```python
from build123d import *

# Parameters (mm, degrees)
ESQUISSE1_W              = 120
ESQUISSE1_H              = 160
BOSS_EXTRU_1_DEPTH       = 40
ESQUISSE2_W              = 110
ESQUISSE2_H              = 150
ENL_V_MAT_EXTRU_1_DEPTH  = 35
CONG_1_R                 = 10
CONG_2_R                 = 10
CONG_3_R                 = 10
ESQUISSE3_R              = 2.5
BOSS_EXTRU_2_DEPTH       = 2.5
CONG_4_R                 = 2.5
ESQUISSE4_R              = 3
ENL_V_MAT_EXTRU_2_DEPTH  = 35
ESQUISSE5_W              = 11
ESQUISSE5_H              = 52
ENL_V_MAT_EXTRU_3_DEPTH  = 2
ESQUISSE6_W              = 52
ESQUISSE6_H              = 11
ENL_V_MAT_EXTRU_4_DEPTH  = 2
ESQUISSE8_W              = 22
ESQUISSE8_H              = 27
ENL_V_MAT_EXTRU_6_DEPTH  = 5
ESQUISSE10_R             = 1
ENL_V_MAT_EXTRU_7_DEPTH  = 4
ESQUISSE11_W             = 10
ESQUISSE11_H             = 10
ENL_V_MAT_EXTRU_8_DEPTH  = 201.062490237
ESQUISSE12_W             = 10
ESQUISSE12_H             = 5.85
ENL_V_MAT_EXTRU_9_DEPTH  = 3
ESQUISSE13_W             = 22
ESQUISSE13_H             = 27
ENL_V_MAT_EXTRU_10_DEPTH = 1
ESQUISSE14_R             = 1
ENL_V_MAT_EXTRU_11_DEPTH = 6
ESQUISSE15_R             = 5
ENL_V_MAT_EXTRU_12_DEPTH = 197.979694385
ESQUISSE16_W             = 22
ESQUISSE16_H             = 17
ENL_V_MAT_EXTRU_13_DEPTH = 2
ESQUISSE17_W             = 26
ESQUISSE17_H             = 22
ENL_V_MAT_EXTRU_14_DEPTH = 2
ESQUISSE18_W             = 26
ESQUISSE18_H             = 22
ENL_V_MAT_EXTRU_15_DEPTH = 2


with BuildPart() as part:
    # Esquisse1 → Boss.-Extru.1 (new body)
    with BuildSketch(Plane(origin=(0, 0, 0), x_dir=(1, 0, 0), z_dir=(0, 1, 0))):
        with Locations((60, 80)):
            Rectangle(ESQUISSE1_W, ESQUISSE1_H)
    extrude(amount=BOSS_EXTRU_1_DEPTH)

    # Esquisse2 → Enlèv. mat.-Extru.1 (cut)
    with BuildSketch(Plane(origin=(0, 40, 0), x_dir=(1, 0, 0), z_dir=(0, 1, 0))):
        with Locations((65, 75)):
            Rectangle(ESQUISSE2_W, ESQUISSE2_H)
    extrude(amount=-ENL_V_MAT_EXTRU_1_DEPTH, mode=Mode.SUBTRACT)

    # Congé1
    cong_1_edges = [part.edges().sort_by_distance(p)[0] for p in [
        (60, 0, -160),
    ]]
    fillet(cong_1_edges, radius=CONG_1_R)

    # Congé2
    cong_2_edges = [part.edges().sort_by_distance(p)[0] for p in [
        (0, 0, -75),
        (0, 2.928932188, -157.071067812),
        (0, 25, -160),
    ]]
    fillet(cong_2_edges, radius=CONG_2_R)

    # Congé3
    cong_3_edges = [part.edges().sort_by_distance(p)[0] for p in [
        (10, 22.5, -150),
    ]]
    fillet(cong_3_edges, radius=CONG_3_R)

    # Esquisse3 → Boss.-Extru.2 (add)
    with BuildSketch(Plane.XZ):
        with Locations(Location((30, -130, 0), (0, 0, 270))):
            Circle(ESQUISSE3_R)
    extrude(amount=BOSS_EXTRU_2_DEPTH)

    # Congé4
    cong_4_edges = [part.edges().sort_by_distance(p)[0] for p in [
        (30, -2.5, -127.5),
    ]]
    fillet(cong_4_edges, radius=CONG_4_R - 0.0001)  # a hair under: the kernel refuses the full size

    # Esquisse4 → Enlèv. mat.-Extru.2 (cut)
    with BuildSketch(Plane(origin=(0, 40, 0), x_dir=(1, 0, 0), z_dir=(0, 1, 0))):
        with Locations(Location((8, 152, 0), (0, 0, 270))):
            Circle(ESQUISSE4_R)
    extrude(amount=-ENL_V_MAT_EXTRU_2_DEPTH, mode=Mode.SUBTRACT)

    # Esquisse5 → Enlèv. mat.-Extru.3 (cut)
    with BuildSketch(Plane(origin=(0, 5, 0), x_dir=(1, 0, 0), z_dir=(0, 1, 0))):
        with Locations((114.5, 75)):
            Rectangle(ESQUISSE5_W, ESQUISSE5_H)
    extrude(amount=-ENL_V_MAT_EXTRU_3_DEPTH, mode=Mode.SUBTRACT)

    # Esquisse6 → Enlèv. mat.-Extru.4 (cut)
    with BuildSketch(Plane(origin=(0, 5, 0), x_dir=(1, 0, 0), z_dir=(0, 1, 0))):
        with Locations((65, 5.5)):
            Rectangle(ESQUISSE6_W, ESQUISSE6_H)
    extrude(amount=-ENL_V_MAT_EXTRU_4_DEPTH, mode=Mode.SUBTRACT)

    # Esquisse8 → Enlèv. mat.-Extru.6 (cut)
    with BuildSketch(Plane.XY.offset(-150)):
        with Locations((41, 22.5)):
            Rectangle(ESQUISSE8_W, ESQUISSE8_H)
    extrude(amount=-ENL_V_MAT_EXTRU_6_DEPTH, mode=Mode.SUBTRACT)

    # Esquisse10 → Enlèv. mat.-Extru.7 (cut)
    with BuildSketch(Plane.XY.offset(-155)):
        with Locations((41, 32.75)):
            Circle(ESQUISSE10_R)
        with Locations((41, 12.25)):
            Circle(ESQUISSE10_R)
    extrude(amount=-ENL_V_MAT_EXTRU_7_DEPTH, mode=Mode.SUBTRACT)

    # Esquisse11 → Enlèv. mat.-Extru.8 (cut, through all)
    with BuildSketch(Plane.XY.offset(-155)):
        with Locations((41, 25.75)):
            Rectangle(ESQUISSE11_W, ESQUISSE11_H)
    extrude(amount=-ENL_V_MAT_EXTRU_8_DEPTH, mode=Mode.SUBTRACT)

    # Esquisse12 → Enlèv. mat.-Extru.9 (cut)
    with BuildSketch(Plane.XY.offset(-155)):
        with Locations((41, 17.825)):
            Rectangle(ESQUISSE12_W, ESQUISSE12_H)
    extrude(amount=-ENL_V_MAT_EXTRU_9_DEPTH, mode=Mode.SUBTRACT)

    # Esquisse13 → Enlèv. mat.-Extru.10 (cut)
    with BuildSketch(Plane.XY.offset(-150)):
        with Locations((78, 22.5)):
            Rectangle(ESQUISSE13_W, ESQUISSE13_H)
    extrude(amount=-ENL_V_MAT_EXTRU_10_DEPTH, mode=Mode.SUBTRACT)

    # Esquisse14 → Enlèv. mat.-Extru.11 (cut)
    with BuildSketch(Plane.XY.offset(-151)):
        with Locations((78, 32.5)):
            Circle(ESQUISSE14_R)
        with Locations((78, 12.5)):
            Circle(ESQUISSE14_R)
    extrude(amount=-ENL_V_MAT_EXTRU_11_DEPTH, mode=Mode.SUBTRACT)

    # Esquisse15 → Enlèv. mat.-Extru.12 (cut, through all)
    with BuildSketch(Plane.XY.offset(-151)):
        with Locations((78, 22.5)):
            Circle(ESQUISSE15_R)
    extrude(amount=-ENL_V_MAT_EXTRU_12_DEPTH, mode=Mode.SUBTRACT)

    # Esquisse16 → Enlèv. mat.-Extru.13 (cut)
    with BuildSketch(Plane.XY.offset(-151)):
        with Locations((78, 22.5)):
            Rectangle(ESQUISSE16_W, ESQUISSE16_H)
    extrude(amount=-ENL_V_MAT_EXTRU_13_DEPTH, mode=Mode.SUBTRACT)

    # Esquisse17 → Enlèv. mat.-Extru.14 (cut)
    with BuildSketch(Plane.XY.offset(-150)):
        with Locations((107, 22.5)):
            Rectangle(ESQUISSE17_W, ESQUISSE17_H)
    extrude(amount=-ENL_V_MAT_EXTRU_14_DEPTH, mode=Mode.SUBTRACT)

    # Esquisse18 → Enlèv. mat.-Extru.15 (cut)
    with BuildSketch(Plane(origin=(10, 0, 0), x_dir=(0, 0, -1), z_dir=(1, 0, 0))):
        with Locations((13, 22.5)):
            Rectangle(ESQUISSE18_W, ESQUISSE18_H)
    extrude(amount=-ENL_V_MAT_EXTRU_15_DEPTH, mode=Mode.SUBTRACT)


solid = part.part
```
Can you work these out from the model? Positions are in its coordinate system, mm. A direction names the side the tool comes from. Round coordinates to 2 decimals unless told otherwise and drop trailing zeros. Order: outer loops, then holes, each group sorted by start corner. A loop starts at its lowest first (then second) coordinate and runs counter-clockwise, first axis right, second up. Notation, with made-up numbers: (-39, 77) -> (-5, 77) arc R28 cw to (-5, 95) -> close; hole circle Ø3 at (23, -1). An arc over 180 degrees is marked (long way). Return JSON: item names as keys, results as strings. Group by question number.
1. If we section it at A-A, the plane y = 22.5: Count the separate pieces of the cut face and the enclosed holes in it, then the cut area to 3 significant figures.
2. We'd pull the mould along Z, two halves only. Please class faces 5 (the face through (82.619, 20.585, -156.451)), 6 (the face through (58, 23, -150)), 7 (the face through (8.9, 22.74, -149.14)): released by +Z, released by -Z, zero draft, split by the parting line, or undercut.
3. If we section it at C-C, the plane z = -77: Write out the boundary of the cut face in (x, y), then the cut area to 3 significant figures.
4. Will these pins go through, and if not, where does the flat tip stop? pin 1 (1.6 mm diameter, centred on y = 4, z = -7, fed in from -X); pin 2 (5 mm diameter, centred on x = 18, z = -102.5, fed in from -Y); pin 3 (6.5 mm diameter, centred on x = 41, y = 16.5, fed in from +Z); pin 4 (9 mm diameter, centred on x = 78, y = 22.5, fed in from +Z).
5. Which directions (+Z, -Z, +X, -X, +Y, -Y) give clear straight access to the entire face, cutting with the end or side of a thin tool? Please do faces 1 (the face through (107, 23, -152)), 2 (the face through (46, 24, -157)), 3 (the face through (64, 5, -76)), 4 (the face through (114, 3, -75)).
6. If we section it at B-B, the plane z = -38: Write out the boundary of the cut face in (x, y).
7. I need wall thicknesses on line 1 (Y direction, x = 41, z = -156.85); line 2 (Y direction, x = 78, z = -155.5); line 3 (X direction, y = 35, z = -118.5). Which ranges of each line are inside material? Lowest first, please. Write a range as [from, to].
8. If we section it at D-D, the plane z = -147: Write out the boundary of the cut face in (x, y), then the cut area to 3 significant figures.
Output values:
{
 "1": {"separate pieces": "3", "enclosed holes": "1", "area": "2,270 mm²"},
 "2": {"face 5": "zero draft", "face 6": "released by +Z", "face 7": "undercut"},
 "3": {"outline": "(0, 10) arc R10 ccw to (10, 0) -> (120, 0) -> (120, 3) -> (109, 3) -> (109, 5) -> (10, 5) -> (10, 40) -> (0, 40) -> close", "area": "907 mm²"},
 "4": {"pin 1": "x = 1.46", "pin 2": "y = 0", "pin 3": "z = -155", "pin 4": "through"},
 "5": {"face 1": "+Z, +X", "face 2": "+Z", "face 3": "+Z, +X, +Y", "face 4": "+X, +Y"},
 "6": {"outline": "(0, 10) arc R10 ccw to (10, 0) -> (120, 0) -> (120, 5) -> (10, 5) -> (10, 40) -> (0, 40) -> close"},
 "7": {"line 1": "[2.71, 11.25], [13.25, 14.9], [30.75, 31.75], [33.75, 40]", "line 2": "[1.65, 11.5], [13.5, 17.5], [27.5, 31.5], [33.5, 40]", "line 3": "[0, 10]"},
 "8": {"outline": "(0, 10) arc R10 ccw to (10, 0) -> (120, 0) -> (120, 5) -> (12.86, 5) -> (12.86, 40) -> (0, 40) -> close", "area": "1,030 mm²"}
}
